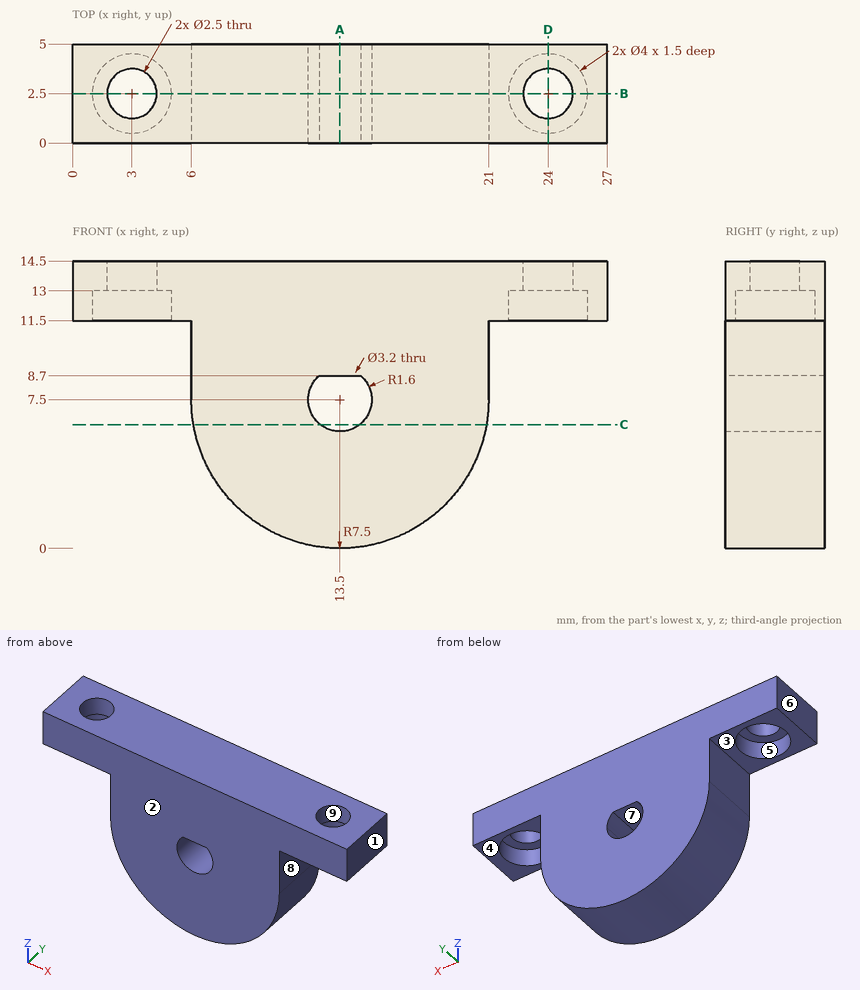
Geometry: see drawing. Coordinates: mm, zero at the bounding-box minimum. A direction names the side the tool comes from. Coordinates: 2 decimals unless noted, no trailing zeros. Write each loop counter-clockwise with the first axis right and the second up, starting at its lowest first coordinate (ties: lowest second). Pieces come first, ordered by that corner, then holes. Notation, with made-up numbers: M 45,10.25 L 81,10.25 A9 ccw 81,16.25 Z; hole C 10,-4.5 d9. An arc over 180 degrees is marked long. Answer as a JSON object with one key per item and string values.
1. Cut plane C-C on z = 6.25. Output: boundary loops of the cut face in (x, y).
Evaluation:
{"outline": "M 6.1,0 L 12.5,0 L 12.5,5 L 6.1,5 Z; M 14.5,0 L 20.9,0 L 20.9,5 L 14.5,5 Z"}
2. Cut plane D-D on x = 24. Output: boundary loops of the cut face in (y, z), plus the area to 3 significant figures.
Evaluation:
{"outline": "M 0,11.5 L 0.5,11.5 L 0.5,13 L 1.25,13 L 1.25,14.5 L 0,14.5 Z; M 3.75,13 L 4.5,13 L 4.5,11.5 L 5,11.5 L 5,14.5 L 3.75,14.5 Z", "area": "5.25 mm^2"}
3. Draft query along X for the marked faces 6, 7, 8 and 9. Return one class per face: released by +X, released by -X, zero draft, split by the parting line, or undercut.
Evaluation:
{"face 6": "released by -X", "face 7": "undercut", "face 8": "released by +X", "face 9": "undercut"}
4. Access query for the marked faces 1, 2, 3, 4 and 5. Directions: +Z, -Z, +X, -X, +Y, -Y. A direction counts if a zero-diameter tool reaches every point of the face in a straight line with its end or side. Return the directions, or none.
Evaluation:
{"face 1": "+Z, -Z, +X, +Y, -Y", "face 2": "+Z, -Z, +X, -X, -Y", "face 3": "-Z, -X, +Y, -Y", "face 4": "-Z, +X, +Y, -Y", "face 5": "-Z"}
5. Cut plane B-B on y = 2.5. Output: boundary loops of the cut face in (x, z).
Evaluation:
{"outline": "M 0,11.5 L 1,11.5 L 1,13 L 1.75,13 L 1.75,14.5 L 0,14.5 Z; M 4.25,13 L 5,13 L 5,11.5 L 6,11.5 L 6,7.5 A7.5 ccw 21,7.5 L 21,11.5 L 22,11.5 L 22,13 L 22.75,13 L 22.75,14.5 L 4.25,14.5 Z; M 25.25,13 L 26,13 L 26,11.5 L 27,11.5 L 27,14.5 L 25.25,14.5 Z; hole M 12.44,8.7 A1.6 ccw long 14.56,8.7 Z"}
6. Contact query for flat-ended pins moving along their axis: P1, Ø2, axis at x = 3, y = 2.5, coming from the +Z side; P2, Ø2, axis at x = 2.5, y = 3.5, coming from the -Z side; P3, Ø1, axis at y = 4, z = 9.5, coming from the -X side; P4, Ø1.5, axis at y = 1.5, z = 12.5, coming from the -X side. Output: stop coordinate, or through.
Evaluation:
{"P1": "through", "P2": "z = 11.5", "P3": "x = 6", "P4": "x = 0"}
7. Cut plane A-A on x = 13.5. Output: boundary loops of the cut face in (y, z), plus the area to 3 significant figures.
Evaluation:
{"outline": "M 0,0 L 5,0 L 5,5.9 L 0,5.9 Z; M 0,8.7 L 5,8.7 L 5,14.5 L 0,14.5 Z", "area": "58.5 mm^2"}
8. Ray query, L1, parallel to Y at x = 24, z = 12.65; L2, parallel to X at y = 2.55, z = 12.5; L3, parallel to Z at x = 23, y = 3.3. Return the intervals inside material, ascending.
Evaluation:
{"L1": "0 to 0.5, 4.5 to 5", "L2": "0 to 1, 5 to 22, 26 to 27", "L3": "13 to 14.5"}
